Autodesk Inventor part; units mm, degrees
ref_plane "YZ Plane" through (0, 0, 0) normal (1, 0, 0) x (0, 1, 0)
ref_plane "XZ Plane" through (0, 0, 0) normal (0, 1, 0) x (-1, 0, 0)
ref_plane "XY Plane" through (0, 0, 0) normal (0, 0, 1) x (1, 0, 0)
sketch "Náčrt1" plane through (0, 0, 0) normal (0, 0, 1) x (1, 0, 0)
  line L0 (52.3561, -3.2889) -> (52.7026, -3.258)
  line L1 (52.7026, -3.258) -> (53.8641, -3.1519)
  line L2 (53.8641, -3.1519) -> (55.0221, -3.0436)
  line L3 (55.0221, -3.0436) -> (56.1757, -2.9334)
  line L4 (56.1757, -2.9334) -> (57.324, -2.8213)
  line L5 (57.324, -2.8213) -> (58.466, -2.7076)
  line L6 (58.466, -2.7076) -> (59.6005, -2.5924)
  line L7 (59.6005, -2.5924) -> (60.7266, -2.476)
  line L8 (60.7266, -2.476) -> (61.843, -2.3584)
  line L9 (61.843, -2.3584) -> (62.9485, -2.2399)
  line L10 (62.9485, -2.2399) -> (64.0421, -2.1207)
  line L11 (64.0421, -2.1207) -> (65.124, -2.0008)
  line L12 (65.124, -2.0008) -> (66.1891, -1.8799)
  line L13 (66.1891, -1.8799) -> (67.2379, -1.7589)
  line L14 (67.2379, -1.7589) -> (68.2689, -1.6383)
  line L15 (68.2689, -1.6383) -> (69.2801, -1.5181)
  line L16 (69.2801, -1.5181) -> (70.27, -1.3988)
  line L17 (70.27, -1.3988) -> (71.2363, -1.2806)
  line L18 (71.2363, -1.2806) -> (72.1771, -1.164)
  line L19 (72.1771, -1.164) -> (73.0899, -1.0493)
  line L20 (73.0899, -1.0493) -> (73.972, -0.937)
  line L21 (73.972, -0.937) -> (74.8205, -0.8276)
  line L22 (74.8205, -0.8276) -> (75.6321, -0.7216)
  line L23 (75.6321, -0.7216) -> (76.4028, -0.6198)
  line L24 (76.4028, -0.6198) -> (77.1281, -0.5229)
  line L25 (77.1281, -0.5229) -> (77.8025, -0.4319)
  line L26 (77.8025, -0.4319) -> (78.4188, -0.3479)
  line L27 (78.4188, -0.3479) -> (78.9642, -0.245)
  line L28 (78.9642, -0.245) -> (79.4284, -0.1574)
  line L29 (79.4284, -0.1574) -> (79.7982, -0.1291)
  line L30 (79.7982, -0.1291) -> (80, -0.1136)
  line L31 (52.3786, 3.287) -> (52.7026, 3.2581)
  line L32 (52.7026, 3.2581) -> (53.864, 3.152)
  line L33 (53.864, 3.152) -> (55.022, 3.0437)
  line L34 (55.022, 3.0437) -> (56.1756, 2.9335)
  line L35 (56.1756, 2.9335) -> (57.3239, 2.8214)
  line L36 (57.3239, 2.8214) -> (58.4658, 2.7077)
  line L37 (58.4658, 2.7077) -> (59.6004, 2.5925)
  line L38 (59.6004, 2.5925) -> (60.7264, 2.4761)
  line L39 (60.7264, 2.4761) -> (61.843, 2.3585)
  line L40 (61.843, 2.3585) -> (62.9486, 2.24)
  line L41 (62.9486, 2.24) -> (64.0421, 2.1208)
  line L42 (64.0421, 2.1208) -> (65.124, 2.0009)
  line L43 (65.124, 2.0009) -> (66.1891, 1.88)
  line L44 (66.1891, 1.88) -> (67.238, 1.759)
  line L45 (67.238, 1.759) -> (68.2689, 1.6383)
  line L46 (68.2689, 1.6383) -> (69.2801, 1.5182)
  line L47 (69.2801, 1.5182) -> (70.27, 1.3989)
  line L48 (70.27, 1.3989) -> (71.2364, 1.2807)
  line L49 (71.2364, 1.2807) -> (72.1771, 1.1641)
  line L50 (72.1771, 1.1641) -> (73.0899, 1.0494)
  line L51 (73.0899, 1.0494) -> (73.972, 0.937)
  line L52 (73.972, 0.937) -> (74.8205, 0.8276)
  line L53 (74.8205, 0.8276) -> (75.6321, 0.7217)
  line L54 (75.6321, 0.7217) -> (76.4028, 0.6199)
  line L55 (76.4028, 0.6199) -> (77.1281, 0.523)
  line L56 (77.1281, 0.523) -> (77.8025, 0.432)
  line L57 (77.8025, 0.432) -> (78.4188, 0.348)
  line L58 (78.4188, 0.348) -> (78.9679, 0.2725)
  line L59 (78.9679, 0.2725) -> (79.4365, 0.208)
  line L60 (79.4365, 0.208) -> (79.8021, 0.1566)
  line L61 (79.8021, 0.1566) -> (80, 0.1287)
  line L62 (80, 0.1287) -> (80, -0.1136)
  line L63 (49.176, -1.5573) -> (50.2021, -1.4704)
  line L64 (50.2021, -1.4704) -> (51.3632, -1.3695)
  line L65 (51.3632, -1.3695) -> (52.5228, -1.2661)
  line L66 (52.5228, -1.2661) -> (53.68, -1.1604)
  line L67 (53.68, -1.1604) -> (54.8339, -1.0525)
  line L68 (54.8339, -1.0525) -> (55.9835, -0.9426)
  line L69 (55.9835, -0.9426) -> (57.1278, -0.831)
  line L70 (57.1278, -0.831) -> (58.2659, -0.7176)
  line L71 (58.2659, -0.7176) -> (59.3966, -0.6029)
  line L72 (59.3966, -0.6029) -> (60.519, -0.4868)
  line L73 (60.519, -0.4868) -> (61.6317, -0.3696)
  line L74 (61.6317, -0.3696) -> (62.7336, -0.2515)
  line L75 (62.7336, -0.2515) -> (63.8236, -0.1327)
  line L76 (63.8236, -0.1327) -> (65.0211, 0)
  line L77 (65.0211, 0) -> (63.8236, 0.1327)
  line L78 (63.8236, 0.1327) -> (62.7337, 0.2516)
  line L79 (62.7337, 0.2516) -> (61.6317, 0.3697)
  line L80 (61.6317, 0.3697) -> (60.5188, 0.4869)
  line L81 (60.5188, 0.4869) -> (59.3965, 0.6029)
  line L82 (59.3965, 0.6029) -> (58.2657, 0.7177)
  line L83 (58.2657, 0.7177) -> (57.1277, 0.831)
  line L84 (57.1277, 0.831) -> (55.9833, 0.9427)
  line L85 (55.9833, 0.9427) -> (54.8338, 1.0526)
  line L86 (54.8338, 1.0526) -> (53.6799, 1.1604)
  line L87 (53.6799, 1.1604) -> (52.5228, 1.2662)
  line L88 (52.5228, 1.2662) -> (51.3632, 1.3696)
  line L89 (51.3632, 1.3696) -> (50.2021, 1.4705)
  line L90 (50.2021, 1.4705) -> (49.0403, 1.5688)
  arc A0 (52.3786, 3.287) -> (52.401, -3.2849) centre (52.0854, 0) ccw
  dimension "d10" = 3.3
extrude "Vysunutí1" add sketch "Náčrt1" along normal mid plane 200
sketch "Náčrt2" plane through (76.4028, 0.6199, 100) normal (0.1324, 0.9912, 0) x (0.9912, -0.1324, 0)
  circle A0 centre (-6.3695, 112.5) radius 1.5
  line L0 (3.6305, 200) -> (3.6305, 0)
  circle A1 centre (-6.3695, 112.5) radius 5
  point P0 (-75.6482, 100)
  point P1 (3.6305, 100)
  dimension "d14" = 3
  dimension "d15" = 12.5
  dimension "d17" = 10
  dimension "d23" = 10
extrude "Vysunutí6" cut sketch "Náčrt2" along normal through all both and the other way through all contours A0
sketch "Náčrt4" plane through (0, 0, 100) normal (0, 0, 1) x (1, 0, 0)
  arc A0 (52.3786, 3.287) -> (52.3561, -3.2889) centre (52.0854, 0) ccw
  circle A1 centre (52.0854, 0) radius 2
  circle A2 centre (57.0854, 0) radius 1.5
  point P0 (0, 0)
  dimension "d31" = 4
  dimension "d32" = 3
  dimension "d33" = 5
extrude "Vysunutí7" [suppressed]
properties part number "horizontal_stab_elevator"
Here's how the part is built. I have some questions about the finished solid (model axes, mm). Coordinates: 2 decimals unless noted, no trailing zeros. Answer as a JSON object with one key per item and string values. Group by question number.
(1) For pin 1 (3 mm diameter, centred on x = 71, y = -2.5, fed in from +Z); pin 2 (1 mm diameter, centred on x = 63.5, z = 37, fed in from -Y); pin 3 (1.5 mm diameter, centred on y = -1, z = -51, fed in from -X); pin 4 (4 mm diameter, centred on x = 58, z = 72.5, fed in from +Y), each with a flat end and sliding along its axis, tell me the tip position at first contact or that it passes through.
(2) I need wall thicknesses on probe 1 along Y at (x, z) = (63, -36.5); probe 2 along Y at (x, z) = (57.5, 15). Which ranges of each line are inside material? Lowest first, please.
(3) If we mould it in two halves opening along Z, with no side actions, what happens to faces 1 (the face through (61, 0, -100)), 2 (the face through (68.384, 0.015, -12.566)), 3 (the face through (48.786, -0.065, -1.4)), 4 (the face through (61, 0, 100))? For each: released by +Z, released by -Z, zero draft, split by the parting line, or undercut.
Values found:
{
 "1": {"pin 1": "stops at z = 100", "pin 2": "stops at y = -2.23", "pin 3": "stops at x = 48.79", "pin 4": "stops at y = 2.95"},
 "2": {"probe 1": "y = -2.23 to 2.23", "probe 2": "y = -2.8 to 2.8"},
 "3": {"face 1": "released by -Z", "face 2": "undercut", "face 3": "zero draft", "face 4": "released by +Z"}
}
